Can you work these out from the model? Positions are in its coordinate system, mm. A direction names the side the tool comes from. Give positions to 0.01 mm unless a question says otherwise; leave off trailing zeros. Write each loop counter-clockwise with the first axis right and the second up, starting at its lowest first coordinate (ties: lowest second). Pieces come first, ordered by that corner, then holes. Notation, with made-up numbers: (-36.75, 88.5) -> (-3.75, 88.5) arc R37 cw to (-3.75, 127.5) -> close; hole circle Ø6 at (-6.75, 0). An arc over 180 degrees is marked (long way). One line per item, written item: value.
Autodesk Inventor part; units mm, degrees
ref_plane "YZ Plane" through (0, 0, 0) normal (1, 0, 0) x (0, 1, 0)
ref_plane "XZ Plane" through (0, 0, 0) normal (0, 1, 0) x (-1, 0, 0)
ref_plane "XY Plane" through (0, 0, 0) normal (0, 0, 1) x (1, 0, 0)
sketch "Sketch1" plane through (0, 0, 0) normal (0, 0, 1) x (1, 0, 0)
  circle A0 centre (0, 0) radius 15 construction
  line L0 (0, 0) -> (-12.9904, 7.5) construction
  line L1 (0, 0) -> (12.9904, 7.5) construction
  line L2 (0, 0) -> (0, -15) construction
  circle A1 centre (-12.9904, 7.5) radius 1.45
  circle A2 centre (12.9904, 7.5) radius 1.45
  circle A3 centre (0, -15) radius 1.45
  circle A4 centre (0, 0) radius 3 construction
  circle A5 centre (0, 0) radius 19
  dimension "d0" = 120
  dimension "d1" = 120
  dimension "d2" = 120
  dimension "d3" = 2.9
  dimension "d4" = 6
  dimension "d5" = 15
  dimension "d6" = 30
  dimension "d7" = 38
extrude "Extrusion1" add sketch "Sketch1" against normal blind 10
sketch "Sketch2" plane through (0, 0, -10) normal (0, 0, -1) x (-1, 0, 0)
  circle A0 centre (0, 0) radius 19
extrude "Extrusion2" add sketch "Sketch2" along normal blind 25.25
fillet "Fillet1" radius 3 1 edges at (19, 0, -35.25)
sketch "Sketch3" plane through (0, 0, 0) normal (0, 0, 1) x (1, 0, 0)
  circle A0 centre (0, 0) radius 19
  circle A1 centre (0, 0) radius 10
  dimension "d13" = 20
extrude "Extrusion3" add sketch "Sketch3" along normal blind 5 contours A1
sketch "Sketch4" plane through (0, 0, 5) normal (0, 0, 1) x (1, 0, 0)
  circle A0 centre (0, 0) radius 10
  circle A1 centre (0, 0) radius 3
  dimension "d16" = 6
extrude "Extrusion4" add sketch "Sketch4" along normal blind 12 contours A1
equation "\"d1\" = d0"
properties part number "rotary encoder"
1) I need wall thicknesses on L1, parallel to X at y = 7, z = -4; L2, parallel to Y at x = 0, z = -2.75; L3, parallel to Z at x = 2, y = -14.5. Which ranges of each line are inside material? Lowest first, please.
Answer list:
L1: x = -17.66 to -14.35, -11.63 to 11.63, 14.35 to 17.66
L2: y = -19 to -16.45, -13.55 to 19
L3: z = -35.25 to 0
2) If we section it at B-B (y = 0): Write out the boundary of the cut face in (x, z), and give its area (3 significant figures).
Answer list:
outline: (-19, -32.25) arc R3 ccw to (-16, -35.25) -> (16, -35.25) arc R3 ccw to (19, -32.25) -> (19, 0) -> (10, 0) -> (10, 5) -> (3, 5) -> (3, 17) -> (-3, 17) -> (-3, 5) -> (-10, 5) -> (-10, 0) -> (-19, 0) -> close
area: 1,510 mm^2
3) If we section it at A-A (x = 0): Write out the boundary of the cut face in (y, z).
Answer list:
outline: (-19, -32.25) arc R3 ccw to (-16, -35.25) -> (16, -35.25) arc R3 ccw to (19, -32.25) -> (19, 0) -> (10, 0) -> (10, 5) -> (3, 5) -> (3, 17) -> (-3, 17) -> (-3, 5) -> (-10, 5) -> (-10, 0) -> (-13.55, 0) -> (-13.55, -10) -> (-16.45, -10) -> (-16.45, 0) -> (-19, 0) -> close
4) Will these pins go through, and if not, where does the flat tip stop? pin 1 (4.5 mm diameter, centred on x = -12.99, y = 7.5, fed in from +Z); pin 2 (3 mm diameter, centred on x = -1.5, z = 2.5, fed in from -Y); pin 3 (1.4 mm diameter, centred on x = -0.5, y = -15.5, fed in from +Z).
Answer list:
pin 1: stops at z = 0
pin 2: stops at y = -10
pin 3: stops at z = -10
5) For faces 4 (the face through (0, 0, 17)), 5 (the face through (-13, 8, -10)), which set-ups out of +Z, -Z, +X, -X, +Y, -Y let a thin tool reach every point of the face, with its end or its side?
Answer list:
face 4: +Z, +X, -X, +Y, -Y
face 5: +Z
6) We'd pull the mould along Y, two halves only. Please class faces 1 (the face through (8, -8, 0)), 2 (the face through (-14.141, 6.618, -4.93)), 3 (the face through (-2.17, 9.76, 2.46)): released by +Y, released by -Y, zero draft, split by the parting line, or undercut.
Answer list:
face 1: zero draft
face 2: undercut
face 3: split by the parting line
7) If we section it at C-C (z = 13): Write out the boundary of the cut face in (x, y), and give its area (3 significant figures).
Answer list:
outline: circle Ø6 at (0, 0)
area: 28.3 mm^2
